Geometry check sheet. Reference: the model listing, model coordinates, mm. Face numbers are marked on the shaded views. Coordinates: 2 decimals unless noted, no trailing zeros. Write each loop counter-clockwise with the first axis right and the second up, starting at its lowest first coordinate (ties: lowest second). Pieces come first, ordered by that corner, then holes. Notation, with made-up numbers: (-4.75, 32.5) -> (16.25, 32.5) arc R25 cw to (16.25, 50.5) -> close; hole circle Ø2 at (-0.75, 73). An arc over 180 degrees is marked (long way). Answer as CSV lines item,"result".
```python
from build123d import *

# Parameters (mm, degrees)
SKETCH_1_R          = 26.8
SKETCH_1_R_2        = 4
SKETCH_1_R_3        = 1.48
SKETCH_1_R_4        = 1.5
EXTRUDE_1_DEPTH     = 3
SKETCH_2_R          = 3
SKETCH_2_R_2        = 1.5
EXTRUDE_2_DEPTH     = 6.9
SKETCH_3_R          = 3
CUT_EXTRUDE_1_DEPTH = 2


with BuildPart() as part:
    # 草图1 → 凸台-拉伸1 (new body)
    with BuildSketch(Plane(origin=(0, 0, 0), x_dir=(1, 0, 0), z_dir=(0, 1, 0))):
        with Locations(Location((0, 0, 0), (0, 0, 270))):
            Circle(SKETCH_1_R)
        with Locations(Location((0, 0, 0), (0, 0, 270))):
            Circle(SKETCH_1_R_2, mode=Mode.SUBTRACT)
        with Locations(Location((0, 7, 0), (0, 0, 270))):
            Circle(SKETCH_1_R_3, mode=Mode.SUBTRACT)
        with Locations(Location((0, 20, 0), (0, 0, 270))):
            Circle(SKETCH_1_R_4, mode=Mode.SUBTRACT)
        with Locations(Location((0, -7, 0), (0, 0, 270))):
            Circle(SKETCH_1_R_3, mode=Mode.SUBTRACT)
        with Locations(Location((7, 0, 0), (0, 0, 270))):
            Circle(SKETCH_1_R_3, mode=Mode.SUBTRACT)
        with Locations(Location((20, 0, 0), (0, 0, 270))):
            Circle(SKETCH_1_R_4, mode=Mode.SUBTRACT)
        with Locations(Location((0, -20, 0), (0, 0, 270))):
            Circle(SKETCH_1_R_4, mode=Mode.SUBTRACT)
        with Locations(Location((-20, 0, 0), (0, 0, 270))):
            Circle(SKETCH_1_R_4, mode=Mode.SUBTRACT)
        with Locations(Location((-7, 0, 0), (0, 0, 270))):
            Circle(SKETCH_1_R_3, mode=Mode.SUBTRACT)
    extrude(amount=EXTRUDE_1_DEPTH)

    # 草图2 → 凸台-拉伸2 (add)
    # profile 1 of 4: a face of its own
    with BuildSketch(Plane(origin=(0, 3, 0), x_dir=(1, 0, 0), z_dir=(0, 1, 0))):
        with Locations(Location((0, 20, 0), (0, 0, 90))):
            Circle(SKETCH_2_R)
        with Locations(Location((0, 20, 0), (0, 0, 270))):
            Circle(SKETCH_2_R_2, mode=Mode.SUBTRACT)
    # profile 2 of 4: a face of its own
    with BuildSketch(Plane(origin=(0, 3, 0), x_dir=(1, 0, 0), z_dir=(0, 1, 0))):
        with Locations(Location((-20, 0, 0), (0, 0, 90))):
            Circle(SKETCH_2_R)
        with Locations(Location((-20, 0, 0), (0, 0, 270))):
            Circle(SKETCH_2_R_2, mode=Mode.SUBTRACT)
    # profile 3 of 4: a face of its own
    with BuildSketch(Plane(origin=(0, 3, 0), x_dir=(1, 0, 0), z_dir=(0, 1, 0))):
        with Locations(Location((20, 0, 0), (0, 0, 90))):
            Circle(SKETCH_2_R)
        with Locations(Location((20, 0, 0), (0, 0, 270))):
            Circle(SKETCH_2_R_2, mode=Mode.SUBTRACT)
    # profile 4 of 4: a face of its own
    with BuildSketch(Plane(origin=(0, 3, 0), x_dir=(1, 0, 0), z_dir=(0, 1, 0))):
        with Locations(Location((0, -20, 0), (0, 0, 90))):
            Circle(SKETCH_2_R)
        with Locations(Location((0, -20, 0), (0, 0, 270))):
            Circle(SKETCH_2_R_2, mode=Mode.SUBTRACT)
    extrude(amount=EXTRUDE_2_DEPTH)

    # 草图3 → 切除-拉伸1 (cut)
    with BuildSketch(Plane.XZ):
        with Locations(Location((0, 20, 0), (0, 0, 270))):
            Circle(SKETCH_3_R)
        with Locations(Location((-20, 0, 0), (0, 0, 270))):
            Circle(SKETCH_3_R)
        with Locations(Location((0, -20, 0), (0, 0, 270))):
            Circle(SKETCH_3_R)
        with Locations(Location((20, 0, 0), (0, 0, 270))):
            Circle(SKETCH_3_R)
    extrude(amount=-CUT_EXTRUDE_1_DEPTH, mode=Mode.SUBTRACT)


solid = part.part
```
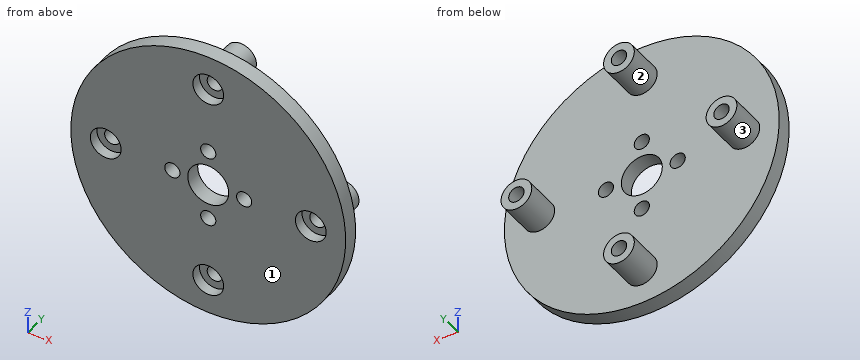
Item 1: Depth check by flat-ended pin: pin 1 Ø8 at (x, z) = (-15.5, -16.5) entering from +Y; pin 2 Ø5 at (y, z) = (5, 19) entering from +X; pin 3 Ø1.8 at (x, z) = (-20, 0) entering from -Y; pin 4 Ø3 at (x, y) = (20.5, 7) entering from -Z. Enter the tip coordinate at first touch or a pass-through.
Responses:
pin 1,"stops at y = 3"
pin 2,"stops at x = 20.3"
pin 3,"passes through"
pin 4,"stops at z = -3"
Item 2: Thickness scan on probe 1 along X at (y, z) = (0.75, 0); probe 2 along Z at (x, y) = (-20, 6.5). Record the ranges inside material, lowest first.
Responses:
probe 1,"x = -26.8 to -23, -17 to -8.48, -5.52 to -4, 4 to 5.52, 8.48 to 17, 23 to 26.8"
probe 2,"z = -3 to -1.5, 1.5 to 3"
Item 3: Cross-section at A-A, the plane y = 8. Record the cut outline in (x, z).
Responses:
outline,"circle Ø6 at (-20, 0); circle Ø6 at (0, -20); circle Ø6 at (0, 20); circle Ø6 at (20, 0); hole circle Ø3 at (-20, 0); hole circle Ø3 at (0, -20); hole circle Ø3 at (0, 20); hole circle Ø3 at (20, 0)"
Item 4: Release check for a two-part mould opening along X. For the marked faces 1, 2 and 3 record: +X half, -X half, draft (parallel to the pull), parting line (faces both ways), or undercut.
Responses:
face 1,"draft"
face 2,"parting line"
face 3,"undercut"
Item 5: Cross-section at C-C, the plane z = 20. Record the cut outline in (x, y), plus the area to 3 significant figures.
Responses:
outline,"(-17.84, 0) -> (-3, 0) -> (-3, 2) -> (-1.5, 2) -> (-1.5, 9.9) -> (-3, 9.9) -> (-3, 3) -> (-17.84, 3) -> close; (1.5, 2) -> (3, 2) -> (3, 0) -> (17.84, 0) -> (17.84, 3) -> (3, 3) -> (3, 9.9) -> (1.5, 9.9) -> close"
area,"113 mm2"
Item 6: Cross-section at D-D, the plane x = 0. Count the separate pieces of the cut face and the enclosed holes in it, plus the area to 3 significant figures.
Responses:
separate pieces,"6"
enclosed holes,"0"
area,"130 mm2"
Item 7: Cross-section at B-B, the plane x = -7. Record the cut outline in (y, z).
Responses:
outline,"(0, -25.87) -> (3, -25.87) -> (3, -1.48) -> (0, -1.48) -> close; (0, 1.48) -> (3, 1.48) -> (3, 25.87) -> (0, 25.87) -> close"
